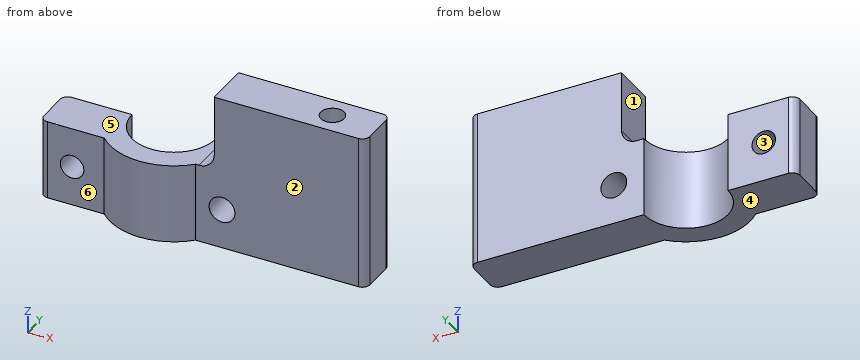
from build123d import *

# Parameters (mm, degrees)
EXTRUDE_1_DEPTH     = 10.5
SKETCH_2_R          = 1.55
CUT_EXTRUDE_1_DEPTH = 31.959651161
SKETCH_3_R          = 1.70728631
CUT_EXTRUDE_2_DEPTH = 31.959651161
SKETCH_5_W          = 20
SKETCH_5_H          = 6
EXTRUDE_2_DEPTH     = 10
SKETCH_6_R          = 1.55
CUT_EXTRUDE_4_DEPTH = 10
FILLET_1_R          = 2
FILLET_2_R          = 1


with BuildPart() as part:
    # 草图1 → 凸台-拉伸1 (new body)
    with BuildSketch(Plane.XY):
        with BuildLine():
            ThreePointArc((-6.020797289, -6), (-7.855786942, -3.246014713), (-8.5, 0))
            Line((-8.5, 0), (-14.5, 0))
            Line((-14.5, 0), (-14.5, -6))
            Line((-14.5, -6), (-6.020797289, -6))
        make_face()
        with BuildLine():
            Line((-8.5, 0), (-5.55, 0))
            ThreePointArc((-5.55, 0), (0, -5.55), (5.55, 0))
            Line((5.55, 0), (8.5, 0))
            ThreePointArc((8.5, 0), (0, -8.5), (-8.5, 0))
        make_face()
        with BuildLine():
            ThreePointArc((8.5, 0), (7.855786942, -3.246014713), (6.020797289, -6))
            Line((6.020797289, -6), (28.5, -6))
            Line((28.5, -6), (28.5, 0))
            Line((28.5, 0), (8.5, 0))
        make_face()
    extrude(amount=EXTRUDE_1_DEPTH)

    # 草图2 → 切除-拉伸1 (cut, through all)
    with BuildSketch(Plane.XZ.offset(6)):
        with Locations(Location((-10.260398645, 5.25, 0), (0, 0, 270))):
            Circle(SKETCH_2_R)
    extrude(amount=-CUT_EXTRUDE_1_DEPTH, mode=Mode.SUBTRACT)

    # 草图3 → 切除-拉伸2 (cut, through all)
    with BuildSketch(Plane.XZ.offset(6)):
        with Locations((9.520797289, 5.25)):
            Circle(SKETCH_3_R)
    extrude(amount=-CUT_EXTRUDE_2_DEPTH, mode=Mode.SUBTRACT)

    # 草图5 → 凸台-拉伸2 (add)
    with BuildSketch(Plane.XY.offset(10.5)):
        with Locations((18.5, -3)):
            Rectangle(SKETCH_5_W, SKETCH_5_H)
    extrude(amount=EXTRUDE_2_DEPTH)

    # 草图6 → 切除-拉伸4 (cut)
    with BuildSketch(Plane.XY.offset(20.5)):
        with Locations((22.5, -3)):
            Circle(SKETCH_6_R)
    extrude(amount=-CUT_EXTRUDE_4_DEPTH, mode=Mode.SUBTRACT)

    # 圆角1
    fillet_1_edges = [part.edges().sort_by_distance(p)[0] for p in [
        (8.5, -3, 10.5),
    ]]
    fillet(fillet_1_edges, radius=FILLET_1_R)

    # 圆角2
    fillet_2_edges = [part.edges().sort_by_distance(p)[0] for p in [
        (-14.5, -6, 5.25),
        (-14.5, 0, 5.25),
        (28.5, 0, 10.25),
        (28.5, -6, 10.25),
    ]]
    fillet(fillet_2_edges, radius=FILLET_2_R)


solid = part.part
Verification items for the finished model (mm, model axes). Face numbers are marked on the shaded views. A direction names the side the tool comes from. Give positions to 0.01 mm unless a question says otherwise; leave off trailing zeros. Order: outer loops, then holes, each group sorted by start corner. A loop starts at its lowest first (then second) coordinate and runs counter-clockwise, first axis right, second up. Notation, with made-up numbers: (37.25, 21) -> (44.25, 21) arc R11 cw to (44.25, 26) -> close; hole circle Ø3 at (-2.75, 35). An arc over 180 degrees is marked (long way). Answer as CSV lines item,"result".
Q1. Depth check by flat-ended pin: pin 1 (2 mm diameter, centred on x = -9, z = 7, fed in from -Y); pin 2 (1.8 mm diameter, centred on y = -2.5, z = 14.5, fed in from -X); pin 3 (0.9 mm diameter, centred on x = 22, y = -3, fed in from +Z). Enter the tip coordinate at first touch or a pass-through.
Solutions:
pin 1,"stops at y = -6"
pin 2,"stops at x = 8.5"
pin 3,"stops at z = 10.5"
Q2. Release check for a two-part mould opening along X. For the marked faces 1, 2 and 3 record: +X half, -X half, draft (parallel to the pull), parting line (faces both ways), or undercut.
Solutions:
face 1,"-X half"
face 2,"draft"
face 3,"undercut"
Q3. Scan lines: probe 1 along X at (y, z) = (-4.5, 4); probe 2 along Y at (x, z) = (26.5, 7.75); probe 3 along X at (y, z) = (-4.5, 2.75). Record each from-to range of solid material in increasing order.
Solutions:
probe 1,"x = -14.5 to -11.18, -9.34 to -3.25, 3.25 to 8.36, 10.68 to 28.5"
probe 2,"y = -6 to 0"
probe 3,"x = -14.5 to -3.25, 3.25 to 28.5"
Q4. Sectioned sample at B-B on z = 15.25. Record the cut outline in (x, y), plus the area to 3 significant figures.
Solutions:
outline,"(8.5, -6) -> (27.5, -6) arc R1 ccw to (28.5, -5) -> (28.5, -1) arc R1 ccw to (27.5, 0) -> (8.5, 0) -> close; hole circle Ø3.1 at (22.5, -3)"
area,"112 mm²"
Q5. Sectioned sample at D-D on z = 2. Record the cut outline in (x, y).
Solutions:
outline,"(-14.5, -5) arc R1 ccw to (-13.5, -6) -> (-6.02, -6) arc R8.5 ccw to (6.02, -6) -> (27.5, -6) arc R1 ccw to (28.5, -5) -> (28.5, -1) arc R1 ccw to (27.5, 0) -> (5.55, 0) arc R5.55 cw to (-5.55, 0) -> (-13.5, 0) arc R1 ccw to (-14.5, -1) -> close"
Q6. Access from +Z, -Z, +X, -X, +Y, -Y to the whole of each face (thin tool, end or side, straight path). Record for the marked faces 4, 5 and 6.
Solutions:
face 4,"-Z, +X, -X, +Y, -Y"
face 5,"+Z, -X, +Y, -Y"
face 6,"+Z, -Z, -X, -Y"
Q7. Sectioned sample at C-C on x = 22.5. Record the cut outline in (y, z).
Solutions:
outline,"(-6, 0) -> (0, 0) -> (0, 20.5) -> (-1.45, 20.5) -> (-1.45, 10.5) -> (-4.55, 10.5) -> (-4.55, 20.5) -> (-6, 20.5) -> close"
Q8. Sectioned sample at A-A on z = 5.25. Record the cut outline in (x, y), plus the area to 3 significant figures.
Solutions:
outline,"(-14.5, -5) arc R1 ccw to (-13.5, -6) -> (-11.81, -6) -> (-11.81, 0) -> (-13.5, 0) arc R1 ccw to (-14.5, -1) -> close; (-8.71, -6) -> (-6.02, -6) arc R8.5 ccw to (6.02, -6) -> (7.81, -6) -> (7.81, 0) -> (5.55, 0) arc R5.55 cw to (-5.55, 0) -> (-8.71, 0) -> close; (11.23, -6) -> (27.5, -6) arc R1 ccw to (28.5, -5) -> (28.5, -1) arc R1 ccw to (27.5, 0) -> (11.23, 0) -> close"
area,"190 mm²"
